Can you work these out from the model? Positions are in its coordinate system, mm. A direction names the side the tool comes from. Give positions to 0.01 mm unless a question says otherwise; leave off trailing zeros. Order: outer loops, then holes, each group sorted by start corner. A loop starts at its lowest first (then second) coordinate and runs counter-clockwise, first axis right, second up. Notation, with made-up numbers: (13.5, 3.25) - (36.5, 3.25) arc R22 ccw to (36.5, 35.25) - close; hole circle Ø9 at (71, 26). An arc over 180 degrees is marked (long way). Return JSON: item names as keys, results as strings.
```python
from build123d import *

# Parameters (mm, degrees)
SKETCH1_R           = 50
BOSS_EXTRUDE1_DEPTH = 30
SKETCH1_3_R         = 2
BOSS_EXTRUDE2_DEPTH = 4
FILLET2_R           = 2


with BuildPart() as part:
    # Sketch1 → Boss-Extrude1 (new body)
    with BuildSketch(Plane(origin=(0, 0, 0), x_dir=(1, 0, 0), z_dir=(0, 1, 0))):
        with Locations(Location((0, 0, 0), (0, 0, 270))):
            Circle(SKETCH1_R)
    extrude(amount=BOSS_EXTRUDE1_DEPTH)

    # Sketch1_3 → Boss-Extrude2 (add)
    # profile 1 of 4: a face of its own
    with BuildSketch(Plane(origin=(0, 0, 0), x_dir=(1, 0, 0), z_dir=(0, 1, 0))):
        with BuildLine():
            Line((-46.5, 33.823069051), (-46.5, 18.377975949))
            ThreePointArc((-46.5, 18.377975949), (-35.355339059, 35.355339059), (-18.377975949, 46.5))
            Line((-18.377975949, 46.5), (-33.823069051, 46.5))
            ThreePointArc((-33.823069051, 46.5), (-40.658639918, 40.658639918), (-46.5, 33.823069051))
        make_face()
        with Locations(Location((-38.183766184, 38.183766184, 0), (0, 0, 270))):
            Circle(SKETCH1_3_R, mode=Mode.SUBTRACT)
    # profile 2 of 4: a face of its own
    with BuildSketch(Plane(origin=(0, 0, 0), x_dir=(1, 0, 0), z_dir=(0, 1, 0))):
        with BuildLine():
            Line((-33.823069051, -46.5), (-18.377975949, -46.5))
            ThreePointArc((-18.377975949, -46.5), (-35.355339059, -35.355339059), (-46.5, -18.377975949))
            Line((-46.5, -18.377975949), (-46.5, -33.823069051))
            ThreePointArc((-46.5, -33.823069051), (-40.658639918, -40.658639918), (-33.823069051, -46.5))
        make_face()
        with Locations(Location((-38.183766184, -38.183766184, 0), (0, 0, 270))):
            Circle(SKETCH1_3_R, mode=Mode.SUBTRACT)
    # profile 3 of 4: a face of its own
    with BuildSketch(Plane(origin=(0, 0, 0), x_dir=(1, 0, 0), z_dir=(0, 1, 0))):
        with BuildLine():
            ThreePointArc((46.5, -18.377975949), (35.355339059, -35.355339059), (18.377975949, -46.5))
            Line((18.377975949, -46.5), (33.823069051, -46.5))
            ThreePointArc((33.823069051, -46.5), (40.658639918, -40.658639918), (46.5, -33.823069051))
            Line((46.5, -33.823069051), (46.5, -18.377975949))
        make_face()
        with Locations(Location((38.183766184, -38.183766184, 0), (0, 0, 270))):
            Circle(SKETCH1_3_R, mode=Mode.SUBTRACT)
    # profile 4 of 4: a face of its own
    with BuildSketch(Plane(origin=(0, 0, 0), x_dir=(1, 0, 0), z_dir=(0, 1, 0))):
        with BuildLine():
            Line((33.823069051, 46.5), (18.377975949, 46.5))
            ThreePointArc((18.377975949, 46.5), (35.355339059, 35.355339059), (46.5, 18.377975949))
            Line((46.5, 18.377975949), (46.5, 33.823069051))
            ThreePointArc((46.5, 33.823069051), (40.658639918, 40.658639918), (33.823069051, 46.5))
        make_face()
        with Locations(Location((38.183766184, 38.183766184, 0), (0, 0, 270))):
            Circle(SKETCH1_3_R, mode=Mode.SUBTRACT)
    extrude(amount=BOSS_EXTRUDE2_DEPTH)

    # Fillet2
    fillet2_edges = [part.edges().sort_by_distance(p)[0] for p in [
        (0, 30, -50),
    ]]
    fillet(fillet2_edges, radius=FILLET2_R)


solid = part.part
```
1. If I drill on L1, parallel to Y at x = -31.5, z = -39; L2, parallel to X at y = 11.75, z = -34.5; L3, parallel to Z at x = -33, y = 2.25, over which ranges is the centre line in solid material (lowest first)? Write a range as [from, to].
Checks:
{"L1": "[0, 4]", "L2": "[-36.19, 36.19]", "L3": "[-46.5, 46.5]"}
2. For pin 1 Ø2 at (x, z) = (26, -14) entering from -Y; pin 2 Ø4 at (x, y) = (25, 22.5) entering from -Z; pin 3 Ø5 at (x, y) = (-13, 19) entering from +Z; pin 4 Ø1.2 at (y, z) = (1, -25) entering from -X, each with a flat end and sliding along its axis, tell me the tip position at first contact or that it passes through.
Checks:
{"pin 1": "y = 0", "pin 2": "z = -44.4", "pin 3": "z = 48.89", "pin 4": "x = -46.5"}
3. Suppose I cut it at A-A (y = 2.25). List the corners of the cut face in (x, z) for me, plus the area to 3 significant figures.
Checks:
{"outline": "(-46.5, -33.82) arc R57.5 ccw to (-33.82, -46.5) - (-18.38, -46.5) arc R50 ccw to (18.38, -46.5) - (33.82, -46.5) arc R57.5 ccw to (46.5, -33.82) - (46.5, -18.38) arc R50 ccw to (46.5, 18.38) - (46.5, 33.82) arc R57.5 ccw to (33.82, 46.5) - (18.38, 46.5) arc R50 ccw to (-18.38, 46.5) - (-33.82, 46.5) arc R57.5 ccw to (-46.5, 33.82) - (-46.5, 18.38) arc R50 ccw to (-46.5, -18.38) - close; hole circle Ø4 at (-38.18, -38.18); hole circle Ø4 at (-38.18, 38.18); hole circle Ø4 at (38.18, -38.18); hole circle Ø4 at (38.18, 38.18)", "area": "8,660 mm^2"}
4. Thinking about a two-plate mould opening in Z: for faces 1 (the face through (37.418, 1.972, -36.336)), 2 (the face through (40.569, 1.972, 40.748)), 3 (the face through (46.5, 2, 26)), which applies, +Z half, -Z half, draft (parallel to the pull), parting line (faces both ways), or undercut?
Checks:
{"face 1": "undercut", "face 2": "+Z half", "face 3": "draft"}
5. On a 3-axis mill with a long thin cutter (end or side, diameter ignored), from which of +Z, -Z, +X, -X, +Y, -Y can I reach the whole of each face in a straight line? I mean faces 4 (the face through (35, 4, -37)), 5 (the face through (46.5, 2, -26)), 6 (the face through (-36.7, 4, 36.5)), 7 (the face through (-37, 4, -36)). Say none if no direction works.
Checks:
{"face 4": "-Z, +X, +Y", "face 5": "-Z, +X, +Y, -Y", "face 6": "+Z, -X, +Y", "face 7": "-Z, -X, +Y"}
